For this review, take the finished solid that the model builds, in its own axes (mm). A direction names the side the tool comes from. Round coordinates to 2 decimals unless told otherwise and drop trailing zeros. Order: outer loops, then holes, each group sorted by start corner. A loop starts at its lowest first (then second) coordinate and runs counter-clockwise, first axis right, second up. Notation, with made-up numbers: M 83.25,2 L 94.25,2 A12 cw 94.25,23 Z; hole C -2.5,62 d10. An arc over 180 degrees is marked long. Answer as a JSON object with one key per item and string values.
from build123d import *

# Parameters (mm, degrees)
SKETCH4_W           = 217.960426721
SKETCH4_H           = 103.66019812
SKETCH4_R           = 2.2
SKETCH4_R_2         = 0.95
BOSS_EXTRUDE1_DEPTH = 4
SKETCH4_7_W         = 217.960426721
SKETCH4_7_H         = 103.66019812
BOSS_EXTRUDE2_DEPTH = 3
CUT_EXTRUDE1_START  = -3
SKETCH4_8_R         = 2.2
CUT_EXTRUDE1_DEPTH  = 3
BOSS_EXTRUDE3_START = 4
BOSS_EXTRUDE3_DEPTH = 3
BOSS_EXTRUDE4_DEPTH = 217.960426721


with BuildPart() as part:
    # Sketch4 → Boss-Extrude1 (new body)
    with BuildSketch(Plane(origin=(0, 0, 0), x_dir=(1, 0, 0), z_dir=(0, 1, 0))):
        with Locations((106.680213361, 49.53009906)):
            Rectangle(SKETCH4_W, SKETCH4_H)
        with Locations(Location((2.54000508, 2.54000508, 0), (0, 0, 270))):
            Circle(SKETCH4_R, mode=Mode.SUBTRACT)
        with Locations(Location((106.68021336, 2.54000508, 0), (0, 0, 270))):
            Circle(SKETCH4_R, mode=Mode.SUBTRACT)
        Polygon((205.360426721, 91.06019812), (205.360426721, 6.5), (8, 6.5), (8, 11.741046482), (2.686004572, 11.741046482), (2.686004572, 18.741046482), (8, 18.741046482), (8, 34.601092202), (2.686004572, 34.601092202), (2.686004572, 41.601092202), (8, 41.601092202), (8, 57.461137922), (2.686004572, 57.461137922), (2.686004572, 64.461137922), (8, 64.461137922), (8, 80.321183642), (2.686004572, 80.321183642), (2.686004572, 87.321183642), (8, 87.321183642), (8, 91.06019812), align=None, mode=Mode.SUBTRACT)
        with Locations(Location((210.820421641, 2.54000508, 0), (0, 0, 270))):
            Circle(SKETCH4_R, mode=Mode.SUBTRACT)
        with Locations(Location((1.792989586, 95.504191008, 0), (0, 0, 270))):
            Circle(SKETCH4_R_2, mode=Mode.SUBTRACT)
        with BuildLine():
            ThreePointArc((11.003022606, 92.679171958), (10.403022606, 93.279171958), (11.003022606, 93.879171958))
            Line((11.003022606, 93.879171958), (11.992807214, 93.879171958))
            ThreePointArc((11.992807214, 93.879171958), (12.592808272, 93.279171958), (11.992807214, 92.679171958))
            Line((11.992807214, 92.679171958), (11.003022606, 92.679171958))
        make_face(mode=Mode.SUBTRACT)
        with Locations(Location((8.792989586, 95.504191008, 0), (0, 0, 270))):
            Circle(SKETCH4_R_2, mode=Mode.SUBTRACT)
        with BuildLine():
            ThreePointArc((2.993222758, 97.129182542), (2.393222758, 97.729182542), (2.993222758, 98.329182542))
            Line((2.993222758, 98.329182542), (3.992807214, 98.329182542))
            ThreePointArc((3.992807214, 98.329182542), (4.592807214, 97.729182542), (3.992807214, 97.129182542))
            Line((3.992807214, 97.129182542), (2.993222758, 97.129182542))
        make_face(mode=Mode.SUBTRACT)
        with BuildLine():
            ThreePointArc((6.093221234, 97.129182542), (5.493221234, 97.729182542), (6.093221234, 98.329182542))
            Line((6.093221234, 98.329182542), (7.09280569, 98.329182542))
            ThreePointArc((7.09280569, 98.329182542), (7.69280569, 97.729182542), (7.09280569, 97.129182542))
            Line((7.09280569, 97.129182542), (6.093221234, 97.129182542))
        make_face(mode=Mode.SUBTRACT)
        with BuildLine():
            ThreePointArc((10.093221234, 97.129182542), (9.493221234, 97.729182542), (10.093221234, 98.329182542))
            Line((10.093221234, 98.329182542), (11.09280569, 98.329182542))
            ThreePointArc((11.09280569, 98.329182542), (11.69280569, 97.729182542), (11.09280569, 97.129182542))
            Line((11.09280569, 97.129182542), (10.093221234, 97.129182542))
        make_face(mode=Mode.SUBTRACT)
        with Locations(Location((27.94005588, 96.52019304, 0), (0, 0, 270))):
            Circle(SKETCH4_R, mode=Mode.SUBTRACT)
        with BuildLine():
            ThreePointArc((206.267621031, 59.659133435), (205.667621031, 60.259133435), (206.267621031, 60.859133435))
            Line((206.267621031, 60.859133435), (207.267205486, 60.859133435))
            ThreePointArc((207.267205486, 60.859133435), (207.867205486, 60.259133435), (207.267205486, 59.659133435))
            Line((207.267205486, 59.659133435), (206.267621031, 59.659133435))
        make_face(mode=Mode.SUBTRACT)
        with BuildLine():
            ThreePointArc((209.367619507, 59.659133435), (208.767619507, 60.259133435), (209.367619507, 60.859133435))
            Line((209.367619507, 60.859133435), (210.367203962, 60.859133435))
            ThreePointArc((210.367203962, 60.859133435), (210.967203962, 60.259133435), (210.367203962, 59.659133435))
            Line((210.367203962, 59.659133435), (209.367619507, 59.659133435))
        make_face(mode=Mode.SUBTRACT)
        with Locations(Location((211.567437135, 62.484124968, 0), (0, 0, 270))):
            Circle(SKETCH4_R_2, mode=Mode.SUBTRACT)
        with Locations(Location((210.820421641, 96.52019304, 0), (0, 0, 270))):
            Circle(SKETCH4_R, mode=Mode.SUBTRACT)
    extrude(amount=BOSS_EXTRUDE1_DEPTH)

    # Sketch4<7> → Boss-Extrude2 (add)
    with BuildSketch(Plane(origin=(0, 0, 0), x_dir=(1, 0, 0), z_dir=(0, 1, 0))):
        with Locations((106.680213361, 49.53009906)):
            Rectangle(SKETCH4_7_W, SKETCH4_7_H)
    extrude(amount=-BOSS_EXTRUDE2_DEPTH)

    # Sketch4<8> → Cut-Extrude1 (cut)
    with BuildSketch(Plane(origin=(0, 0, 0), x_dir=(1, 0, 0), z_dir=(0, 1, 0)).offset(CUT_EXTRUDE1_START)):
        with Locations(Location((27.94005588, 96.52019304, 0), (0, 0, 270))):
            Circle(SKETCH4_8_R)
        with Locations(Location((210.820421641, 96.52019304, 0), (0, 0, 270))):
            Circle(SKETCH4_8_R)
        with Locations(Location((210.820421641, 2.54000508, 0), (0, 0, 270))):
            Circle(SKETCH4_8_R)
        with Locations(Location((106.68021336, 2.54000508, 0), (0, 0, 270))):
            Circle(SKETCH4_8_R)
        with Locations(Location((2.54000508, 2.54000508, 0), (0, 0, 270))):
            Circle(SKETCH4_8_R)
    extrude(amount=CUT_EXTRUDE1_DEPTH, mode=Mode.SUBTRACT)

    # Sketch4<10> → Boss-Extrude3 (add)
    with BuildSketch(Plane(origin=(0, 0, 0), x_dir=(1, 0, 0), z_dir=(0, 1, 0)).offset(BOSS_EXTRUDE3_START)):
        Polygon((-0.3, -0.3), (-0.3, 92.987071374), (-2.3, 92.987071374), (-2.3, -2.3), (215.660426721, -2.3), (215.660426721, 59.944119888), (213.660426721, 59.944119888), (213.660426721, -0.3), align=None)
        Polygon((-0.3, 99.36019812), (192.548387097, 99.36019812), (192.548387097, 101.36019812), (-2.3, 101.36019812), (-2.3, 98.044196088), (-0.3, 98.044196088), align=None)
        Polygon((202.168402337, 101.36019812), (202.168402337, 99.36019812), (213.660426721, 99.36019812), (213.660426721, 65.001244602), (215.660426721, 65.001244602), (215.660426721, 101.36019812), align=None)
    extrude(amount=BOSS_EXTRUDE3_DEPTH)

    # Sketch5 → Boss-Extrude4 (add)
    with BuildSketch(Plane.ZY.offset(2.3)):
        Polygon((2.3, -3), (-101.36019812, -3), (-101.36019812, -18), align=None)
    extrude(amount=-BOSS_EXTRUDE4_DEPTH)


solid = part.part
1) For L1, parallel to X at y = 1.5, z = -52; L2, parallel to Z at x = 180, y = 1; L3, parallel to Z at x = 76, y = 5.5, list the stretches that pass through material, from the lowest coordinate up.
Geometry check:
{"L1": "x = -2.3 to 8, 205.36 to 215.66", "L2": "z = -101.36 to -91.06, -6.5 to 2.3", "L3": "z = -101.36 to -99.36, 0.3 to 2.3"}
2) Mouldability with a two-part tool opening along Z and no side actions: class faces 1 (the flat face through (8, 2, -27)), 2 (the flat face through (-2.3, -3, -62)), 3 (the flat face through (105, 2, 2.3)), 4 (the flat face through (5, 2, -64.461)) as +Z half, -Z half, draft (parallel to the pull), parting line (faces both ways), or undercut.
Geometry check:
{"face 1": "undercut", "face 2": "draft", "face 3": "+Z half", "face 4": "undercut"}
3) Add section A-A on x = 59.5. State the section outline as (y, z) points, and give its area (3 significant figures).
Geometry check:
{"outline": "M -18,-101.36 L 7,-101.36 L 7,-99.36 L 4,-99.36 L 4,-91.06 L 0,-91.06 L 0,-6.5 L 4,-6.5 L 4,0.3 L 7,0.3 L 7,2.3 L -3,2.3 Z", "area": "1,180 mm²"}
4) Insertion check: P1, Ø5, axis at x = 34.5, z = -39.5, coming from the -Y side; P2, Ø12, axis at x = 55.5, z = -70, coming from the +Y side; P3, Ø5, axis at x = 106.68, z = -2.54, coming from the -Y side. Each pin has a flat end and moves straight along its axis. Give the tip position at first contact, or say it passes through.
Geometry check:
{"P1": "stops at y = -9.41", "P2": "stops at y = 0", "P3": "stops at y = -4.06"}
5) Add section C-C on y = -9.75. State the section outline as (x, z) points, and give its area (3 significant figures).
Geometry check:
{"outline": "M -2.3,-101.36 L 215.66,-101.36 L 215.66,-44.35 L -2.3,-44.35 Z", "area": "12,400 mm²"}
6) Add section B-B on z = -27.5. State the section outline as (x, y) points, and give its area (3 significant figures).
Geometry check:
{"outline": "M -2.3,-7.31 L 215.66,-7.31 L 215.66,7 L 213.66,7 L 213.66,4 L 205.36,4 L 205.36,0 L 8,0 L 8,4 L -0.3,4 L -0.3,7 L -2.3,7 Z", "area": "1,690 mm²"}
7) Machinability: for faces 5 (the flat face through (2.686, 2, -15)), 6 (the flat face through (215.66, -3, -60)), which of the approach directions +Z, -Z, +X, -X, +Y, -Y give a long, thin tool a straight path to every point of the face, cutting with its end or side? Answer none if there is none.
Geometry check:
{"face 5": "+Y", "face 6": "+Z, -Z, +X, +Y, -Y"}
